Geometry: final body of the model. Coordinates: model frame, mm. Give positions to 0.01 mm unless a question says otherwise; leave off trailing zeros. Write each loop counter-clockwise with the first axis right and the second up, starting at its lowest first coordinate (ties: lowest second). Pieces come first, ordered by that corner, then holes. Notation, with made-up numbers: M 39.5,-28.75 L 78.5,-28.75 A28 cw 78.5,-9.75 Z; hole C 22.25,-33 d4. An arc over 180 degrees is marked long. Use a Markdown table: item, result. Add a question column.
(1) Cut plane A-A (z = 105). Output: boundary loops of the cut face in (x, y).
(2) Cut plane C-C (z = -91.5). Output: boundary loops of the cut face in (x, y).
(3) Pin query (flat end, axial travel): pin 1 Ø8.5 at (y, z) = (-10, 165) entering from +X. Return the tip coordinate at first contact, or that it passes through.
(4) Material intervals for L1, parallel to Y at x = 0.5, z = -165; L2, parallel to Z at x = 9.5, y = 2; L3, parallel to X at y = -13, z = 133, sorted ascending.
(5) Cut plane D-D (y = -30). State how many separate pieces and enclosed holes the cut face has, plus the area to 3 significant figures.
(6) Cut plane B-B (y = 22). Output: boundary loops of the cut face in (x, z), plus the area to 3 significant figures.
(7) Draft query along Y for faces 1 (the flat face through (7, 5, -187.263)), 2 (the cylindrical face through (0.65, -9.86, -71.74)), 3 (the flat face through (1, -42, 1)). Return one class per face: released by +Y, released by -Y, zero draft, split by the parting line, or undercut.
```python
from build123d import *

# Parameters (mm, degrees)
SKETCH1_W           = 374.525504892
SKETCH1_H           = 95
SKETCH1_R           = 3.2639
BOSS_EXTRUDE1_DEPTH = 1.31064
SKETCH2_W           = 1.31064
SKETCH2_H           = 95
BOSS_EXTRUDE2_DEPTH = 12.7


with BuildPart() as part:
    # Sketch1 → Boss-Extrude1 (new body)
    with BuildSketch(Plane(origin=(0, 0, 0), x_dir=(0, 0, -1), z_dir=(1, 0, 0))):
        with Locations((0, 5.5)):
            Rectangle(SKETCH1_W, SKETCH1_H)
        with Locations((-165, -30)):
            Circle(SKETCH1_R, mode=Mode.SUBTRACT)
        with Locations((-135, -30)):
            Circle(SKETCH1_R, mode=Mode.SUBTRACT)
        with Locations((-105, -30)):
            Circle(SKETCH1_R, mode=Mode.SUBTRACT)
        with Locations((-75, -30)):
            Circle(SKETCH1_R, mode=Mode.SUBTRACT)
        with Locations((-45, -30)):
            Circle(SKETCH1_R, mode=Mode.SUBTRACT)
        with Locations((-15, -30)):
            Circle(SKETCH1_R, mode=Mode.SUBTRACT)
        with Locations((15, -30)):
            Circle(SKETCH1_R, mode=Mode.SUBTRACT)
        with Locations((45, -30)):
            Circle(SKETCH1_R, mode=Mode.SUBTRACT)
        with Locations((75, -30)):
            Circle(SKETCH1_R, mode=Mode.SUBTRACT)
        with Locations((105, -30)):
            Circle(SKETCH1_R, mode=Mode.SUBTRACT)
        with Locations((135, -30)):
            Circle(SKETCH1_R, mode=Mode.SUBTRACT)
        with Locations((165, -30)):
            Circle(SKETCH1_R, mode=Mode.SUBTRACT)
        with Locations((-135, -10)):
            Circle(SKETCH1_R, mode=Mode.SUBTRACT)
        with Locations((-105, -10)):
            Circle(SKETCH1_R, mode=Mode.SUBTRACT)
        with Locations((-75, -10)):
            Circle(SKETCH1_R, mode=Mode.SUBTRACT)
        with Locations((-45, -10)):
            Circle(SKETCH1_R, mode=Mode.SUBTRACT)
        with Locations((-15, -10)):
            Circle(SKETCH1_R, mode=Mode.SUBTRACT)
        with Locations((15, -10)):
            Circle(SKETCH1_R, mode=Mode.SUBTRACT)
        with Locations((45, -10)):
            Circle(SKETCH1_R, mode=Mode.SUBTRACT)
        with Locations((75, -10)):
            Circle(SKETCH1_R, mode=Mode.SUBTRACT)
        with Locations((105, -10)):
            Circle(SKETCH1_R, mode=Mode.SUBTRACT)
        with Locations((135, -10)):
            Circle(SKETCH1_R, mode=Mode.SUBTRACT)
        with Locations((165, -10)):
            Circle(SKETCH1_R, mode=Mode.SUBTRACT)
        with Locations((-135, 10)):
            Circle(SKETCH1_R, mode=Mode.SUBTRACT)
        with Locations((-105, 10)):
            Circle(SKETCH1_R, mode=Mode.SUBTRACT)
        with Locations((-75, 10)):
            Circle(SKETCH1_R, mode=Mode.SUBTRACT)
        with Locations((-45, 10)):
            Circle(SKETCH1_R, mode=Mode.SUBTRACT)
        with Locations((-15, 10)):
            Circle(SKETCH1_R, mode=Mode.SUBTRACT)
        with Locations((15, 10)):
            Circle(SKETCH1_R, mode=Mode.SUBTRACT)
        with Locations((45, 10)):
            Circle(SKETCH1_R, mode=Mode.SUBTRACT)
        with Locations((75, 10)):
            Circle(SKETCH1_R, mode=Mode.SUBTRACT)
        with Locations((105, 10)):
            Circle(SKETCH1_R, mode=Mode.SUBTRACT)
        with Locations((135, 10)):
            Circle(SKETCH1_R, mode=Mode.SUBTRACT)
        with Locations((165, 10)):
            Circle(SKETCH1_R, mode=Mode.SUBTRACT)
        with Locations((-135, 30)):
            Circle(SKETCH1_R, mode=Mode.SUBTRACT)
        with Locations((-105, 30)):
            Circle(SKETCH1_R, mode=Mode.SUBTRACT)
        with Locations((-75, 30)):
            Circle(SKETCH1_R, mode=Mode.SUBTRACT)
        with Locations((-45, 30)):
            Circle(SKETCH1_R, mode=Mode.SUBTRACT)
        with Locations((-15, 30)):
            Circle(SKETCH1_R, mode=Mode.SUBTRACT)
        with Locations((15, 30)):
            Circle(SKETCH1_R, mode=Mode.SUBTRACT)
        with Locations((45, 30)):
            Circle(SKETCH1_R, mode=Mode.SUBTRACT)
        with Locations((75, 30)):
            Circle(SKETCH1_R, mode=Mode.SUBTRACT)
        with Locations((105, 30)):
            Circle(SKETCH1_R, mode=Mode.SUBTRACT)
        with Locations((135, 30)):
            Circle(SKETCH1_R, mode=Mode.SUBTRACT)
        with Locations((165, 30)):
            Circle(SKETCH1_R, mode=Mode.SUBTRACT)
        with Locations((-165, -10)):
            Circle(SKETCH1_R, mode=Mode.SUBTRACT)
        with Locations((-165, 10)):
            Circle(SKETCH1_R, mode=Mode.SUBTRACT)
        with Locations((-165, 30)):
            Circle(SKETCH1_R, mode=Mode.SUBTRACT)
    extrude(amount=BOSS_EXTRUDE1_DEPTH)

    # Sketch2 → Boss-Extrude2 (add)
    with BuildSketch(Plane(origin=(1.31064, 0, 0), x_dir=(0, 0, -1), z_dir=(1, 0, 0))):
        with Locations((-186.607432446, 5.5)):
            Rectangle(SKETCH2_W, SKETCH2_H)
        with Locations((186.607432446, 5.5)):
            Rectangle(SKETCH2_W, SKETCH2_H)
    extrude(amount=BOSS_EXTRUDE2_DEPTH)


solid = part.part
```
Answer list:
| question | item | result |
|---|---|---|
| 1 | outline | M 0,-42 L 1.31,-42 L 1.31,-33.26 L 0,-33.26 Z; M 0,-26.74 L 1.31,-26.74 L 1.31,-13.26 L 0,-13.26 Z; M 0,-6.74 L 1.31,-6.74 L 1.31,6.74 L 0,6.74 Z; M 0,13.26 L 1.31,13.26 L 1.31,26.74 L 0,26.74 Z; M 0,33.26 L 1.31,33.26 L 1.31,53 L 0,53 Z |
| 2 | outline | M 0,-42 L 1.31,-42 L 1.31,53 L 0,53 Z |
| 3 | pin 1 | x = 1.31 |
| 4 | L1 | -42 to -33.26, -26.74 to -13.26, -6.74 to 6.74, 13.26 to 26.74, 33.26 to 53 |
| 4 | L2 | -187.26 to -185.95, 185.95 to 187.26 |
| 4 | L3 | 0 to 1.31 |
| 5 | separate pieces | 13 |
| 5 | enclosed holes | 0 |
| 5 | area | 421 mm² |
| 6 | outline | M 0,-187.26 L 14.01,-187.26 L 14.01,-185.95 L 1.31,-185.95 L 1.31,185.95 L 14.01,185.95 L 14.01,187.26 L 0,187.26 Z |
| 6 | area | 524 mm² |
| 7 | face 1 | zero draft |
| 7 | face 2 | undercut |
| 7 | face 3 | released by -Y |
